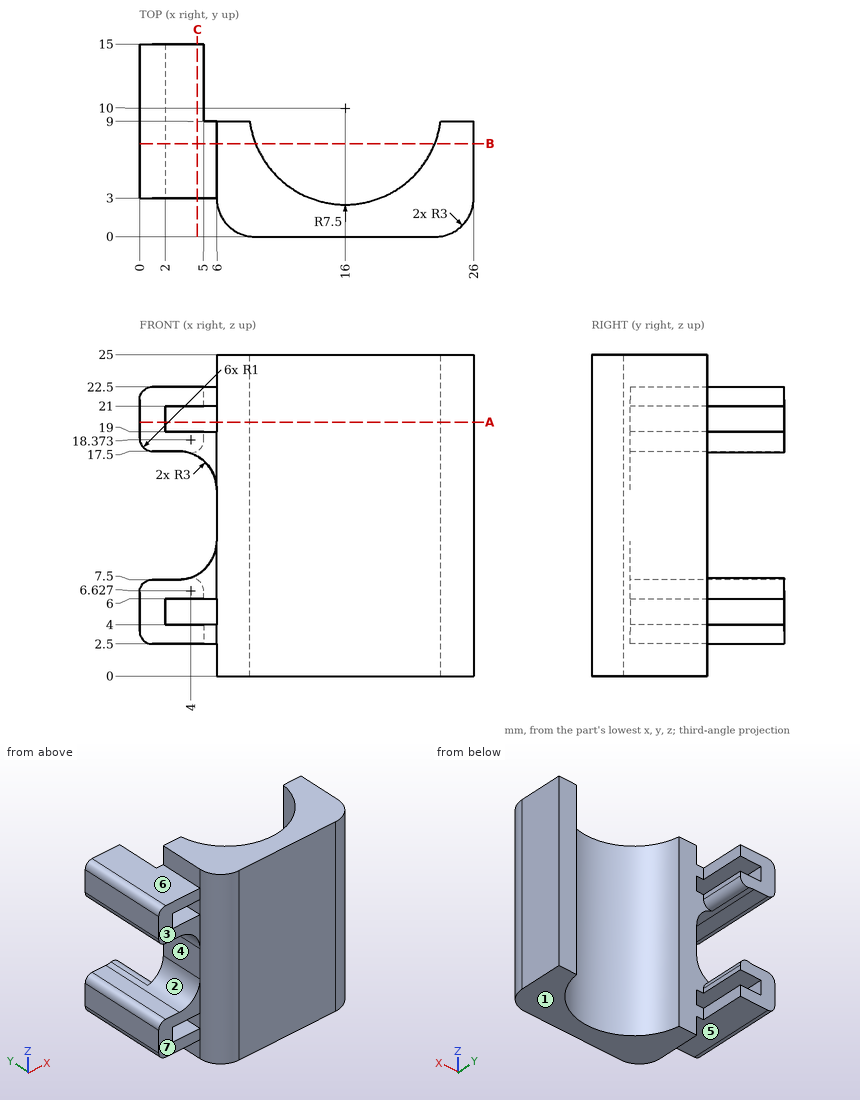
Answer from the drawing. Dimensions are ordinates in mm from the lowest x, y and z of the part. A direction names the side the tool comes from. Give positions to 0.01 mm unless a question says otherwise; leave off trailing zeros. Loops run counter-clockwise (first coordinate to the right, second up) from the corner with the lowest first, then second, coordinate; pieces in that order, holes last. Notation, with made-up numbers: M 39,25 L 86,25 A30 ccw 86,50 Z; hole C 55,76.5 d6. An arc over 180 degrees is marked long. One line per item, written item: value.
Q1. A cutting plane is placed at C-C on x = 4.5. Determine the outline of the cut face in (y, z).
Working result:
outline: M 3,2.5 L 15,2.5 L 15,4 L 3,4 Z; M 3,6 L 15,6 L 15,7.49 L 9,7.49 L 9,7.9 L 3,7.9 Z; M 3,17.1 L 9,17.1 L 9,17.51 L 15,17.51 L 15,19 L 3,19 Z; M 3,21 L 15,21 L 15,22.5 L 3,22.5 Z
Q2. Flat-ended cylindrical pins translate along their axes: P1, Ø0.6, axis at x = 1.5, y = 10.5, coming from the +Z side; P2, Ø1.2, axis at y = 6, z = 11.5, coming from the -X side; P3, Ø0.7, axis at y = 13.5, z = 6.5, coming from the +X side. Find the tip coordinate at first contact, or state that the pin passes through.
Working result:
P1: stops at z = 22.5
P2: stops at x = 6
P3: stops at x = 5
Q3. Determine the mould class of the marked faces 1, 2 and 3 for opening direction Z: +Z half, -Z half, draft (parallel to the pull), parting line (faces both ways), or undercut.
Working result:
face 1: -Z half
face 2: undercut
face 3: draft
Q4. A cutting plane is placed at B-B on y = 7.25. Give the number of separate pieces and of enclosed holes in the cut face, then the cut area to 3 significant figures.
Working result:
separate pieces: 2
enclosed holes: 2
area: 198 mm^2
Q5. A cutting plane is placed at A-A on z = 19.75. Determine the outline of the cut face in (x, y), then the cut area to 3 significant figures.
Working result:
outline: M 0,3 L 2,3 L 2,15 L 0,15 Z; M 6,3 A3 ccw 9,0 L 23,0 A3 ccw 26,3 L 26,9 L 23.43,9 A7.5 cw 8.57,9 L 6,9 Z
area: 127 mm^2
Q6. Find the intervals of material crossed by line 1 (Z direction, x = 1, y = 3.75); line 2 (Z direction, x = 5.5, y = 7); line 3 (X direction, y = 8.25, z = 3), in increasing order. Write a range as from..to.
Working result:
line 1: z = 2.5..7.5, 17.5..22.5
line 2: z = 2.5..4, 6..8.84, 16.16..19, 21..22.5
line 3: x = 0.13..8.71, 23.29..26
Q7. For the marked faces 4, 5, 6 and 7, determine the directions among +Z, -Z, +X, -X, +Y, -Y from which every point of the face is accessible in a straight line to the end or side of a thin tool.
Working result:
face 4: -X, +Y, -Y
face 5: -Z, -X, +Y, -Y
face 6: +Z, -X, +Y, -Y
face 7: +Z, -Z, -X, -Y
